The model under review builds one solid part; all positions refer to its coordinate system, in mm. Face numbers are marked on the shaded views. A direction names the side the tool comes from. Give positions to 0.01 mm unless a question says otherwise; leave off trailing zeros. Order: outer loops, then holes, each group sorted by start corner. A loop starts at its lowest first (then second) coordinate and runs counter-clockwise, first axis right, second up. Notation, with made-up numbers: (22.25, 85.5) -> (59.25, 85.5) arc R23 cw to (59.25, 101.5) -> close; hole circle Ø2 at (6.25, -24). An arc over 180 degrees is marked (long way). Answer as a JSON object with one key per item and string values. Group by question number.
from build123d import *

# Parameters (mm, degrees)
SKETCH1_R           = 1.65
SKETCH1_R_2         = 6.15
BOSS_EXTRUDE1_DEPTH = 72
CUT_EXTRUDE1_DEPTH  = 57
SKETCH3_R           = 1.5
CUT_EXTRUDE2_DEPTH  = 92.028841583
FILLET1_R           = 6


with BuildPart() as part:
    # Sketch1 → Boss-Extrude1 (new body)
    with BuildSketch(Plane.XY):
        with BuildLine():
            Line((-21, 0), (-21, -21.5))
            Line((-21, -21.5), (-36, -21.5))
            Line((-36, -21.5), (-36, -24.5))
            Line((-36, -24.5), (36, -24.5))
            Line((36, -24.5), (36, -21.5))
            Line((36, -21.5), (21, -21.5))
            Line((21, -21.5), (21, 0))
            ThreePointArc((21, 0), (0, 21), (-21, 0))
        make_face()
        with Locations((0, -15.5)):
            Circle(SKETCH1_R, mode=Mode.SUBTRACT)
        with Locations((-13.423393759, -7.75)):
            Circle(SKETCH1_R, mode=Mode.SUBTRACT)
        with Locations((-13.423393759, 7.75)):
            Circle(SKETCH1_R, mode=Mode.SUBTRACT)
        with Locations((0, 15.5)):
            Circle(SKETCH1_R, mode=Mode.SUBTRACT)
        with Locations((13.423393759, 7.75)):
            Circle(SKETCH1_R, mode=Mode.SUBTRACT)
        with Locations((13.423393759, -7.75)):
            Circle(SKETCH1_R, mode=Mode.SUBTRACT)
        with Locations((-7, 0)):
            Circle(SKETCH1_R_2, mode=Mode.SUBTRACT)
    extrude(amount=BOSS_EXTRUDE1_DEPTH)

    # Sketch2 → Cut-Extrude1 (cut)
    with BuildSketch(Plane.XY.offset(72)):
        with BuildLine():
            Line((-18.5, 0), (-18.5, -21.5))
            Line((-18.5, -21.5), (18.5, -21.5))
            Line((18.5, -21.5), (18.5, 0))
            ThreePointArc((18.5, 0), (0, 18.5), (-18.5, 0))
        make_face()
    extrude(amount=-CUT_EXTRUDE1_DEPTH, mode=Mode.SUBTRACT)

    # Sketch3 → Cut-Extrude2 (cut, through all)
    with BuildSketch(Plane(origin=(0, -21.5, 0), x_dir=(1, 0, 0), z_dir=(0, 1, 0))):
        with Locations(Location((-28.5, -36, 0), (0, 0, 270))):
            Circle(SKETCH3_R)
        with Locations(Location((-28.5, -6, 0), (0, 0, 270))):
            Circle(SKETCH3_R)
        with Locations(Location((-28.5, -66, 0), (0, 0, 270))):
            Circle(SKETCH3_R)
        with Locations(Location((28.5, -66, 0), (0, 0, 90))):
            Circle(SKETCH3_R)
        with Locations(Location((28.5, -6, 0), (0, 0, 90))):
            Circle(SKETCH3_R)
        with Locations(Location((28.5, -36, 0), (0, 0, 90))):
            Circle(SKETCH3_R)
    extrude(amount=-CUT_EXTRUDE2_DEPTH, mode=Mode.SUBTRACT)

    # Fillet1
    fillet1_edges = [part.edges().sort_by_distance(p)[0] for p in [
        (-36, -23, 0),
    ]]
    fillet(fillet1_edges, radius=FILLET1_R)


solid = part.part
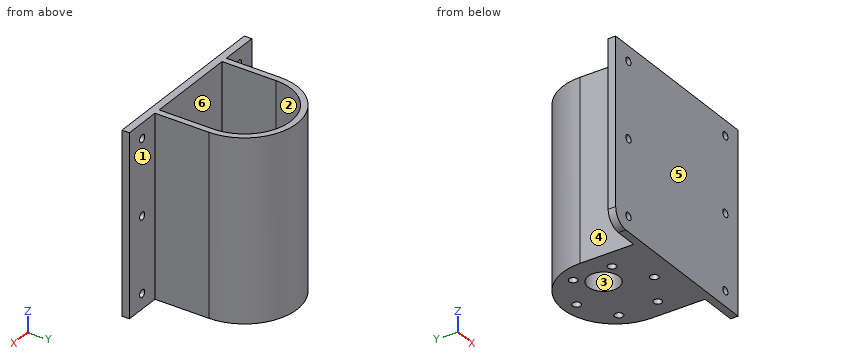
1. Take a section at C-C on z = 16. Give the boundary of the cut face in (x, y).
2. Draft analysis for pull direction X (two halves, no side actions). For the marked faces 4, 5 and 6, state which applies: pulls with the +X half, pulls with the -X half, needs draft (parallel to the pull), parting line crosses it, or undercut.
3. Machinability: for the marked faces 1, 2 and 3, which of the approach directions +Z, -Z, +X, -X, +Y, -Y give a long, thin tool a straight path to every point of the face, cutting with its end or side? Answer none if there is none.
4. For pin 1 (3.5 mm diameter, centred on x = 28.5, z = 66, fed in from +Y); pin 2 (4 mm diameter, centred on x = 13.42, y = -7.75, fed in from +Z); pin 3 (23.5 mm diameter, centred on y = -6, z = 30.5, fed in from +X), all flat-tipped, find the tip position at first contact; note any pin that passes through.
5. Take a section at A-A on x = -28.5. Give the boundary of the cut face in (y, z).
6. Take a section at B-B on y = 7.75. Give the boundary of the cut face in (x, z).
7. For probe 1 along Y at (x, z) = (0, 9.5); probe 2 along X at (y, z) = (-7.75, 11.5); probe 3 along Z at (x, y) = (28.5, -22.4), list the stretches that pass through material, from the lowest coordinate up. Write a range as [from, to].
8. Take a section at D-D on y = -15.5. Give the boundary of the cut face in (x, z), plus the area to 4 significant figures.
Checks:
{
 "1": {"outline": "(-36, -24.5) -> (36, -24.5) -> (36, -21.5) -> (21, -21.5) -> (21, 0) arc R21 ccw to (-21, 0) -> (-21, -21.5) -> (-36, -21.5) -> close; hole (-18.5, -21.5) -> (18.5, -21.5) -> (18.5, 0) arc R18.5 ccw to (-18.5, 0) -> close"},
 "2": {"face 4": "pulls with the -X half", "face 5": "needs draft", "face 6": "undercut"},
 "3": {"face 1": "+Z, -Z, +X, +Y", "face 2": "+Z", "face 3": "+Z, -Z"},
 "4": {"pin 1": "stops at y = -21.5", "pin 2": "stops at z = 15", "pin 3": "stops at x = 21"},
 "5": {"outline": "(-24.5, 0) -> (-21.5, 0) -> (-21.5, 4.5) -> (-24.5, 4.5) -> close; (-24.5, 7.5) -> (-21.5, 7.5) -> (-21.5, 34.5) -> (-24.5, 34.5) -> close; (-24.5, 37.5) -> (-21.5, 37.5) -> (-21.5, 64.5) -> (-24.5, 64.5) -> close; (-24.5, 67.5) -> (-21.5, 67.5) -> (-21.5, 72) -> (-24.5, 72) -> close"},
 "6": {"outline": "(-19.52, 0) -> (-15.07, 0) -> (-15.07, 15) -> (-16.8, 15) -> (-16.8, 72) -> (-19.52, 72) -> close; (-11.77, 0) -> (11.77, 0) -> (11.77, 15) -> (-11.77, 15) -> close; (15.07, 0) -> (19.52, 0) -> (19.52, 72) -> (16.8, 72) -> (16.8, 15) -> (15.07, 15) -> close"},
 "7": {"probe 1": "y = [-24.5, -17.15], [-13.85, 13.85], [17.15, 21]", "probe 2": "x = [-21, -15.07], [-11.77, 11.77], [15.07, 21]", "probe 3": "z = [0, 4.5], [7.5, 34.5], [37.5, 64.5], [67.5, 72]"},
 "8": {"outline": "(-21, 0) -> (-1.65, 0) -> (-1.65, 15) -> (-18.5, 15) -> (-18.5, 72) -> (-21, 72) -> close; (1.65, 0) -> (21, 0) -> (21, 72) -> (18.5, 72) -> (18.5, 15) -> (1.65, 15) -> close", "area": "865.5 mm2"}
}
